Part model, mm, in its own coordinate system. A direction names the side the tool comes from. Round coordinates to 2 decimals unless told otherwise and drop trailing zeros. Write each loop counter-clockwise with the first axis right and the second up, starting at its lowest first coordinate (ties: lowest second). Pieces come first, ordered by that corner, then holes. Notation, with made-up numbers: (4.5, 74) -> (32.5, 74) arc R13 cw to (32.5, 78) -> close; hole circle Ø1 at (-11, 12). An arc over 180 degrees is marked (long way). Return JSON: item names as keys, results as strings. Group by question number.
(1) Drill centre lines: L1, parallel to X at y = 2.25, z = 41.25; L2, parallel to Z at x = 41, y = 4.25; L3, parallel to X at y = 3.5, z = 27.5. Where is each one in solid material? Low to high. Write a range as from..to.
(2) Saw through at C-C (z = -14). List the corners of the cut face in (x, y).
(3) Saw through at A-A (x = -71.5). List the corners of the cut face in (y, z).
(4) Tool access for faces 1 (the flat face through (-1, 5, 42.25)), 2 (the flat face through (-75.25, 4, 1)): list every direction of +Z, -Z, +X, -X, +Y, -Y with a clear straight run to the whole face (end or side of a thin tool).
(5) Mould opens along Z. For faces 3 (the flat face through (0, 8, -44)), 4 (the cylindrical face through (-69.517, 4.056, -41.51)), 5 (the flat face through (-1, 4, -45.25)) say: +Z half, -Z half, draft (parallel to the pull), parting line (faces both ways), or undercut.
(6) Drop a flat-ended pin along its axis: pin 1 Ø10 at (x, z) = (-45.5, -29.5) entering from +Y. Give the stop position or say it passes through.
(7) Saw through at B-B (y = 6.5). List the corners of the cut face in (x, z), plus the area to 3 significant figures.
(8) Saw through at D-D (x = -28). List the corners of the cut face in (y, z).
from build123d import *

# Parameters (mm, degrees)
SKETCH1_W           = 150.5
SKETCH1_H           = 90.5
SKETCH1_W_2         = 137.5
SKETCH1_H_2         = 84.5
BOSS_EXTRUDE1_DEPTH = 8
SKETCH2_R           = 2
CUT_EXTRUDE1_DEPTH  = 39
SKETCH3_W           = 84.5
SKETCH3_H           = 2.5
BOSS_EXTRUDE2_DEPTH = 138


with BuildPart() as part:
    # Sketch1 → Boss-Extrude1 (new body)
    with BuildSketch(Plane(origin=(0, 0, 0), x_dir=(1, 0, 0), z_dir=(0, 1, 0))):
        Rectangle(SKETCH1_W, SKETCH1_H)
        Rectangle(SKETCH1_W_2, SKETCH1_H_2, mode=Mode.SUBTRACT)
    extrude(amount=BOSS_EXTRUDE1_DEPTH)

    # Sketch2 → Cut-Extrude1 (cut)
    with BuildSketch(Plane(origin=(0, 8, 0), x_dir=(1, 0, 0), z_dir=(0, 1, 0))):
        with Locations(Location((-71.5, 41.25, 0), (0, 0, 270))):
            Circle(SKETCH2_R)
        with Locations(Location((-71.5, -41.25, 0), (0, 0, 270))):
            Circle(SKETCH2_R)
        with Locations(Location((71.5, -41.25, 0), (0, 0, 270))):
            Circle(SKETCH2_R)
        with Locations(Location((71.5, 41.25, 0), (0, 0, 270))):
            Circle(SKETCH2_R)
    extrude(amount=-CUT_EXTRUDE1_DEPTH, mode=Mode.SUBTRACT)

    # Sketch3 → Boss-Extrude2 (add)
    with BuildSketch(Plane(origin=(-68.75, 0, 0), x_dir=(0, 0, -1), z_dir=(1, 0, 0))):
        with Locations((0, 1.25)):
            Rectangle(SKETCH3_W, SKETCH3_H)
    extrude(amount=BOSS_EXTRUDE2_DEPTH)


solid = part.part
Computed values:
{
 "1": {"L1": "-75.25..-73.5, -69.5..69.5, 73.5..75.25", "L2": "-45.25..-42.25, 42.25..45.25", "L3": "-75.25..-68.75, 68.75..75.25"},
 "2": {"outline": "(-75.25, 0) -> (75.25, 0) -> (75.25, 8) -> (68.75, 8) -> (68.75, 2.5) -> (-68.75, 2.5) -> (-68.75, 8) -> (-75.25, 8) -> close"},
 "3": {"outline": "(0, -45.25) -> (8, -45.25) -> (8, -43.25) -> (0, -43.25) -> close; (0, -39.25) -> (8, -39.25) -> (8, 39.25) -> (0, 39.25) -> close; (0, 43.25) -> (8, 43.25) -> (8, 45.25) -> (0, 45.25) -> close"},
 "4": {"face 1": "+Y", "face 2": "+Z, -Z, -X, +Y, -Y"},
 "5": {"face 3": "draft", "face 4": "undercut", "face 5": "-Z half"},
 "6": {"pin 1": "y = 2.5"},
 "7": {"outline": "(-75.25, -45.25) -> (75.25, -45.25) -> (75.25, 45.25) -> (-75.25, 45.25) -> close; hole circle Ø4 at (-71.5, -41.25); hole circle Ø4 at (-71.5, 41.25); hole (-68.75, -42.25) -> (68.75, -42.25) -> (68.75, 42.25) -> (-68.75, 42.25) -> close; hole circle Ø4 at (71.5, -41.25); hole circle Ø4 at (71.5, 41.25)", "area": "1,950 mm2"},
 "8": {"outline": "(0, -45.25) -> (8, -45.25) -> (8, -42.25) -> (2.5, -42.25) -> (2.5, 42.25) -> (8, 42.25) -> (8, 45.25) -> (0, 45.25) -> close"}
}
